from build123d import *

# Parameters (mm, degrees)
BOSS_EXTRUDE1_DEPTH = 44


with BuildPart() as part:
    # Sketch1 → Boss-Extrude1 (new body)
    with BuildSketch(Plane(origin=(0, 0, 0), x_dir=(0, 0, -1), z_dir=(1, 0, 0))):
        with BuildLine():
            ThreePointArc((-24.093171188, 0), (-0.779280479, 14.75), (22.534610231, 0))
            Line((22.534610231, 0), (29.120719521, 0))
            Line((29.120719521, 0), (29.120719521, 1))
            Line((29.120719521, 1), (23.158921208, 1))
            ThreePointArc((23.158921208, 1), (-0.779280479, 15.75), (-24.717482165, 1))
            Line((-24.717482165, 1), (-30.679280479, 1))
            Line((-30.679280479, 1), (-30.679280479, 0))
            Line((-30.679280479, 0), (-24.093171188, 0))
        make_face()
    extrude(amount=BOSS_EXTRUDE1_DEPTH)


solid = part.part
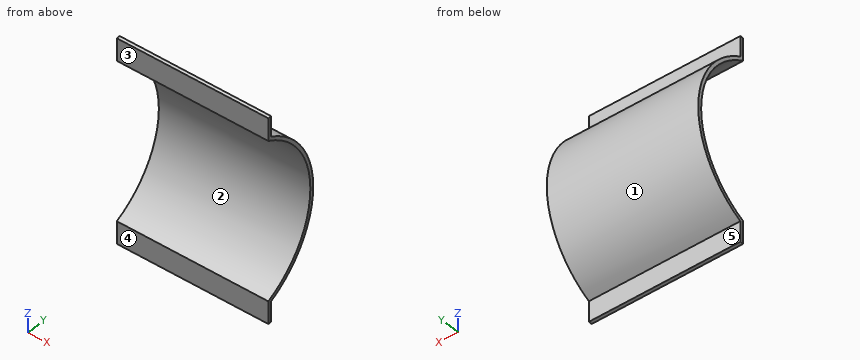
Could you check a few things on this model? Use its own coordinates, in mm. Face numbers are marked on the shaded views. A direction names the side the tool comes from. Give positions to 0.01 mm unless a question says otherwise; leave off trailing zeros. Order: outer loops, then holes, each group sorted by start corner. A loop starts at its lowest first (then second) coordinate and runs counter-clockwise, first axis right, second up. Notation, with made-up numbers: (-25.75, -34.75) - (-10.75, -34.75) arc R17 cw to (-10.75, -25.75) - close; hole circle Ø10 at (76.25, -27). An arc over 180 degrees is marked (long way). Return JSON: item names as keys, results as strings. Group by question number.
Q1. Thinking about a two-plate mould opening in Z: for the marked faces 1, 2 and 3, which applies, pulls with the +Z half, pulls with the -Z half, needs draft (parallel to the pull), parting line crosses it, or undercut?
Q2. Suppose I cut it at A-A, the plane y = 11.75. Please give me the cut outline in (x, z), and give its area (3 significant figures).
Q3. Please list where these lines run through material, in increasing order: line 1 along Y through (x, z) = (28, -25); line 2 along Z through (x, y) = (16.5, 5); line 3 along Z through (x, y) = (3.5, 3). Write a range as [from, to].
Q4. Will these pins go through, and if not, where does the flat tip stop? pin 1 Ø6 at (x, y) = (39, 6.5) entering from -Z; pin 2 Ø5 at (x, y) = (6, 5.5) entering from -Z; pin 3 Ø1.5 at (x, z) = (23, 16) entering from +Y.
Q5. Suppose I cut it at C-C, the plane y = 7. Please give me the cut outline in (x, z).
Q6. Which directions (+Z, -Z, +X, -X, +Y, -Y) give clear straight access to the entire face, cutting with the end or side of a thin tool? Please do the marked faces 4 and 5.
Q7. Suppose I cut it at B-B, the plane x = 34.5. Please give me the cut outline in (y, z), and give its area (3 significant figures).
Q8. Suppose I cut it at D-D, the plane z = 21. Please give me the cut outline in (x, y), and give its area (3 significant figures).
Resolved:
{
 "1": {"face 1": "parting line crosses it", "face 2": "undercut", "face 3": "needs draft"},
 "2": {"outline": "(0, -13.31) - (44, -13.31) - (44, -11.3) - (0, -11.3) - close; (0, 12.85) - (44, 12.85) - (44, 14.86) - (0, 14.86) - close", "area": "177 mm2"},
 "3": {"line 1": "y = [0, 1]", "line 2": "z = [-20.68, -19.42], [20.98, 22.24]", "line 3": "z = [-22.04, -20.86], [22.42, 23.6]"},
 "4": {"pin 1": "stops at z = -21.73", "pin 2": "stops at z = -22.04", "pin 3": "stops at y = 11.51"},
 "5": {"outline": "(0, -19.03) - (44, -19.03) - (44, -17.66) - (0, -17.66) - close; (0, 19.21) - (44, 19.21) - (44, 20.59) - (0, 20.59) - close"},
 "6": {"face 4": "+Z, -Z, +X, -X, -Y", "face 5": "-Z, +X, -X, +Y"},
 "7": {"outline": "(0, -29.12) - (1, -29.12) - (1, -23.16) arc R26.8 ccw to (1, 24.72) - (1, 30.68) - (0, 30.68) - (0, 24.09) arc R25.8 cw to (0, -22.53) - close", "area": "71.3 mm2"},
 "8": {"outline": "(0, 4.97) - (44, 4.97) - (44, 6.54) - (0, 6.54) - close", "area": "68.9 mm2"}
}
